from build123d import *

# Parameters (mm, degrees)
SKETCH1_R           = 4.05765
SKETCH1_R_2         = 3.5306
SKETCH1_R_3         = 2.032
SKETCH1_R_4         = 1.6002
BOSS_EXTRUDE1_DEPTH = 3.175
SKETCH1_7_R         = 1.6002
CUT_EXTRUDE4_DEPTH  = 0.9525
SKETCH3_W           = 1.27
SKETCH3_H           = 1.905
FILLET1_R           = 0.635
FILLET2_R           = 0.635


with BuildPart() as part:
    # Sketch1 → Boss-Extrude1 (new, symmetric)
    with BuildSketch(Plane.XY):
        with BuildLine():
            Line((7.14375, 31.75), (7.14375, 0))
            ThreePointArc((7.14375, 0), (0, -7.14375), (-7.14375, 0))
            Line((-7.14375, 0), (-7.14375, 31.75))
            Line((-7.14375, 31.75), (7.14375, 31.75))
        make_face()
        Circle(SKETCH1_R, mode=Mode.SUBTRACT)
        with Locations((0, 19.05)):
            Circle(SKETCH1_R_2, mode=Mode.SUBTRACT)
        with Locations((-3.96875, 28.575)):
            Circle(SKETCH1_R_3, mode=Mode.SUBTRACT)
        with Locations((3.96875, 28.575)):
            Circle(SKETCH1_R_3, mode=Mode.SUBTRACT)
        with Locations((4.60375, 9.525)):
            Circle(SKETCH1_R_4, mode=Mode.SUBTRACT)
    extrude(amount=BOSS_EXTRUDE1_DEPTH, both=True)

    # Sketch1<7> → Cut-Extrude4 (cut, symmetric)
    with BuildSketch(Plane.XY):
        with BuildLine():
            Line((7.14375, 6.6548), (7.14375, 12.3952))
            Line((7.14375, 12.3952), (4.60375, 12.3952))
            ThreePointArc((4.60375, 12.3952), (1.73355, 9.525), (4.60375, 6.6548))
            Line((4.60375, 6.6548), (7.14375, 6.6548))
        make_face()
        with Locations((4.60375, 9.525)):
            Circle(SKETCH1_7_R, mode=Mode.SUBTRACT)
    extrude(amount=CUT_EXTRUDE4_DEPTH, both=True, mode=Mode.SUBTRACT)

    # Cut-Sweep1: sweep along a path in Sketch2
    with BuildLine(Plane.XY.offset(3.175)) as cut_sweep1_path:
        Line((7.14375, 6.6548), (7.14375, 0))
        ThreePointArc((7.14375, 0), (0, -7.14375), (-7.14375, 0))
        Line((-7.14375, 0), (-7.14375, 6.35))
    # Sketch3 → Cut-Sweep1 (sweep, cut)
    with BuildSketch(Plane(origin=(0, 6.6548, 0), x_dir=(1, 0, 0), z_dir=(0, 1, 0))):
        with Locations((6.50875, 0)):
            Rectangle(SKETCH3_W, SKETCH3_H)
    sweep(path=cut_sweep1_path.line, mode=Mode.SUBTRACT)

    # Fillet1
    fillet1_edges = [part.edges().sort_by_distance(p)[0] for p in [
        (0, -7.14375, 3.175),
        (-7.14375, 15.875, -3.175),
        (0, 31.75, -3.175),
        (7.14375, 15.875, 3.175),
        (7.14375, 15.875, -3.175),
        (0, -7.14375, -3.175),
        (-7.14375, 31.75, 0),
        (7.14375, 31.75, 0),
        (0, 31.75, 3.175),
        (-7.14375, 15.875, 3.175),
    ]]
    fillet(fillet1_edges, radius=FILLET1_R)

    # Fillet2
    fillet2_edges = [part.edges().sort_by_distance(p)[0] for p in [
        (5.87375, 6.6548, 0),
        (7.14375, 12.3952, 0),
        (-7.14375, 6.35, 0),
        (-5.87375, 6.35, 0),
    ]]
    fillet(fillet2_edges, radius=FILLET2_R - 0.0001)  # a hair under: the kernel refuses the full size


solid = part.part
Read the model definition and answer for the solid it produces. Units are mm, in the model's axes. A direction names the side the tool comes from. Give positions to 0.01 mm unless a question says otherwise; leave off trailing zeros. Loops run counter-clockwise (first coordinate to the right, second up) from the corner with the lowest first, then second, coordinate; pieces in that order, holes last. Notation, with made-up numbers: (9, 62) - (53, 62) arc R6 ccw to (53, 66) - close; hole circle Ø4 at (28, -37). An arc over 180 degrees is marked (long way). Answer as CSV lines item,"result". Start each with the question number.
1) Determine the mould class of faces 5 (the face through (-0.88, -3.96, -0.04)), 6 (the face through (5.874, 3, 0)), 7 (the face through (0, 13, -3.175)) for opening direction Z: released by +Z, released by -Z, zero draft, split by the parting line, or undercut.
2) Find section B-B (x = 0). State how many separate pieces and enclosed holes the cut face has, then the cut area to 3 significant figures.
3) Find section C-C (y = 8.5). Write down the section's boundary in (x, z) (1 decimal).
4) Straight lines are drawn through the part: L1, parallel to Y at x = 0, z = -0.5; L2, parallel to Y at x = -1.75, z = 2.5; L3, parallel to Y at x = -3, z = 2.5. For each, find the intervals that lie inside material, in ascending order. Write a range as from..to.
5) Which of the six approach directions +Z, -Z, +X, -X, +Y, -Y give full straight-line access (tool end or side, diameter ignored) to faces 1 (the face through (0.129, -5.872, 0.013)), 2 (the face through (-5.874, 3, 0)), 3 (the face through (6.3, 1.5, -0.952)), 4 (the face through (6, 12.395, 0))?
6) Find section A-A (y = 19.05). Write down the section's boundary in (x, z) (3 decimals), then the cut area to 3 significant figures.
7) Each of these flat-tipped pins is pushed along its axis until it touches: pin 1 Ø0.6 at (y, z) = (1.5, 0) entering from +X; pin 2 Ø1 at (y, z) = (2.5, 0) entering from -X. Where does it stop, or does it pass through?
Findings below:
1,face 5,"zero draft"
1,face 6,"undercut"
1,face 7,"released by -Z"
2,separate pieces,"3"
2,enclosed holes,"0"
2,area,"148 mm^2"
3,outline,"(-7.1, -2.5) arc R0.6 ccw to (-6.5, -3.2) - (3.4, -3.2) - (3.4, -1) - (1.9, -1) - (1.9, 1) - (3.4, 1) - (3.4, 3.2) - (-6.5, 3.2) arc R0.6 ccw to (-7.1, 2.5) - close; (5.8, -3.2) - (6.5, -3.2) arc R0.6 ccw to (7.1, -2.5) - (7.1, -1) - (5.8, -1) - close; (5.8, 1) - (7.1, 1) - (7.1, 2.5) arc R0.6 ccw to (6.5, 3.2) - (5.8, 3.2) - close"
4,L1,"-5.87..-4.06, 4.06..15.52, 22.58..31.75"
4,L2,"-6.93..-3.66, 3.66..15.98, 22.12..31.75"
4,L3,"-6.48..-2.73, 2.73..17.19, 20.91..26.79, 30.36..31.75"
5,face 1,"-Y"
5,face 2,"-X, -Y"
5,face 3,"none"
5,face 4,"+X"
6,outline,"(-7.144, -2.54) arc R0.635 ccw to (-6.509, -3.175) - (-3.531, -3.175) - (-3.531, 3.175) - (-6.509, 3.175) arc R0.635 ccw to (-7.144, 2.54) - close; (3.531, -3.175) - (6.509, -3.175) arc R0.635 ccw to (7.144, -2.54) - (7.144, 2.54) arc R0.635 ccw to (6.509, 3.175) - (3.531, 3.175) - close"
6,area,"45.5 mm^2"
7,pin 1,"x = 5.87"
7,pin 2,"x = -5.87"
